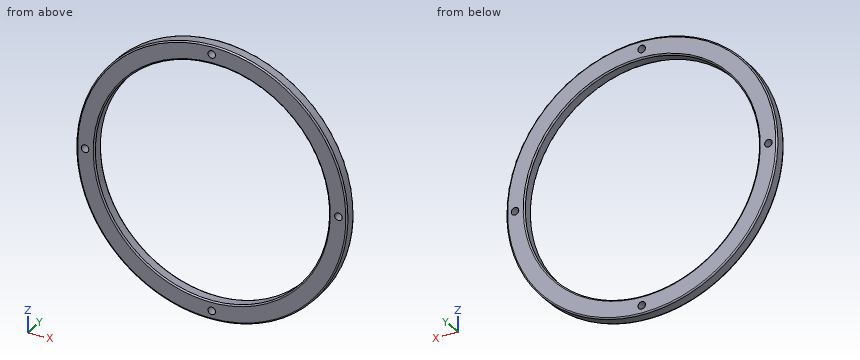
from build123d import *

# Parameters (mm, degrees)
SKETCH1_R           = 100
SKETCH1_R_2         = 86.5
BOSS_EXTRUDE1_DEPTH = 8.5
FILLET1_R           = 1
SKETCH2_R           = 2.75
CUT_EXTRUDE1_DEPTH  = 142.676568423


with BuildPart() as part:
    # Sketch1 → Boss-Extrude1 (new body)
    with BuildSketch(Plane(origin=(0, 0, 0), x_dir=(1, 0, 0), z_dir=(0, 1, 0))):
        with Locations(Location((0, 0, 0), (0, 0, 270))):
            Circle(SKETCH1_R)
        with Locations(Location((0, 0, 0), (0, 0, 270))):
            Circle(SKETCH1_R_2, mode=Mode.SUBTRACT)
    extrude(amount=BOSS_EXTRUDE1_DEPTH)

    # Fillet1
    fillet1_edges = [part.edges().sort_by_distance(p)[0] for p in [
        (0, 0, -100),
        (0, 8.5, -100),
        (0, 0, -86.5),
        (0, 8.5, -86.5),
    ]]
    fillet(fillet1_edges, radius=FILLET1_R)

    # Sketch2 → Cut-Extrude1 (cut, through all)
    with BuildSketch(Plane(origin=(0, 8.5, 0), x_dir=(1, 0, 0), z_dir=(0, 1, 0))):
        with Locations(Location((0, 93.5, 0), (0, 0, 270))):
            Circle(SKETCH2_R)
        with Locations(Location((93.5, 0, 0), (0, 0, 270))):
            Circle(SKETCH2_R)
        with Locations(Location((0, -93.5, 0), (0, 0, 270))):
            Circle(SKETCH2_R)
        with Locations(Location((-93.5, 0, 0), (0, 0, 270))):
            Circle(SKETCH2_R)
    extrude(amount=-CUT_EXTRUDE1_DEPTH, mode=Mode.SUBTRACT)


solid = part.part
The listing builds one solid part. Answer for the finished solid, in the listing's coordinates (mm). Coordinates: 2 decimals unless noted, no trailing zeros. Write each loop counter-clockwise with the first axis right and the second up, starting at its lowest first coordinate (ties: lowest second). Pieces come first, ordered by that corner, then holes. Notation, with made-up numbers: (22, -11.75) -> (52, -11.75) arc R24 ccw to (52, 9.25) -> close; hole circle Ø3 at (-30, -22). An arc over 180 degrees is marked (long way). One line per question, with ' | ' between items.
1. Section B-B (x = 0) is taken. Determine the outline of the cut face in (y, z), and give its area (3 significant figures).
Verdict:
outline: (0, -99) arc R1 ccw to (1, -100) -> (7.5, -100) arc R1 ccw to (8.5, -99) -> (8.5, -96.25) -> (0, -96.25) -> close; (0, -90.75) -> (8.5, -90.75) -> (8.5, -87.5) arc R1 ccw to (7.5, -86.5) -> (1, -86.5) arc R1 ccw to (0, -87.5) -> close; (0, 87.5) arc R1 ccw to (1, 86.5) -> (7.5, 86.5) arc R1 ccw to (8.5, 87.5) -> (8.5, 90.75) -> (0, 90.75) -> close; (0, 96.25) -> (8.5, 96.25) -> (8.5, 99) arc R1 ccw to (7.5, 100) -> (1, 100) arc R1 ccw to (0, 99) -> close | area: 134 mm^2
2. Section C-C (y = 5.75) is taken. Determine the outline of the cut face in (x, z), and give its area (3 significant figures).
Verdict:
outline: circle Ø200 at (0, 0); hole circle Ø5.5 at (-93.5, 0); hole circle Ø173 at (0, 0); hole circle Ø5.5 at (0, -93.5); hole circle Ø5.5 at (0, 93.5); hole circle Ø5.5 at (93.5, 0) | area: 7,810 mm^2
3. Section A-A (z = 0) is taken. Determine the outline of the cut face in (x, y), and give its area (3 significant figures).
Verdict:
outline: (-100, 1) arc R1 ccw to (-99, 0) -> (-96.25, 0) -> (-96.25, 8.5) -> (-99, 8.5) arc R1 ccw to (-100, 7.5) -> close; (-90.75, 0) -> (-87.5, 0) arc R1 ccw to (-86.5, 1) -> (-86.5, 7.5) arc R1 ccw to (-87.5, 8.5) -> (-90.75, 8.5) -> close; (86.5, 1) arc R1 ccw to (87.5, 0) -> (90.75, 0) -> (90.75, 8.5) -> (87.5, 8.5) arc R1 ccw to (86.5, 7.5) -> close; (96.25, 0) -> (99, 0) arc R1 ccw to (100, 1) -> (100, 7.5) arc R1 ccw to (99, 8.5) -> (96.25, 8.5) -> close | area: 134 mm^2
4. Given pin 1 Ø2 at (y, z) = (1.5, 32) entering from -X; pin 2 Ø4 at (y, z) = (3, -9.5) entering from -X; pin 3 Ø1 at (y, z) = (7, 41.5) entering from +X; pin 4 Ø6.5 at (x, z) = (93.5, 0) entering from -Y, each flat-ended and moving along its own axis, determine where each tip first touches the part or whether it passes through.
Verdict:
pin 1: stops at x = -95.07 | pin 2: stops at x = -99.72 | pin 3: stops at x = 91.21 | pin 4: stops at y = 0
5. Straight lines are drawn through the part: line 1 (X direction, y = 6.5, z = 0); line 2 (X direction, y = 2.25, z = 16); line 3 (X direction, y = 7, z = -78.5). For each, find the intervals that lie inside material, in ascending order.
Verdict:
line 1: x = -100 to -96.25, -90.75 to -86.5, 86.5 to 90.75, 96.25 to 100 | line 2: x = -98.71 to -85.01, 85.01 to 98.71 | line 3: x = -61.95 to -36.33, 36.33 to 61.95
